Geometry check sheet. Reference: the model listing, model coordinates, mm. A direction names the side the tool comes from. Round coordinates to 2 decimals unless told otherwise and drop trailing zeros. Write each loop counter-clockwise with the first axis right and the second up, starting at its lowest first coordinate (ties: lowest second). Pieces come first, ordered by that corner, then holes. Notation, with made-up numbers: M 16.25,57 L 46.25,57 A25 cw 46.25,82 Z; hole C -18,1.25 d2. An arc over 180 degrees is marked long. Put each result on its own line as item: value. Start each with the question number.
(1) Gauge pin test, flat ends, axial feed: pin 1 (16.5 mm diameter, centred on x = -35, y = 6.5, fed in from -Z); pin 2 (7.5 mm diameter, centred on x = -35.5, y = 7, fed in from +Z); pin 3 (7.5 mm diameter, centred on y = 7.5, z = -22, fed in from -X). Record the tip position at first contact, or that the pin passes through.
(2) Material ranges on probe 1 along X at (y, z) = (26, -2); probe 2 along X at (y, z) = (12.5, -5); probe 3 along Z at (x, y) = (27, 28), recorded low to high.
(3) Tool access check on faces 1 (the flat face through (53, 7, -59.295)), 2 (the flat face through (-74.848, 27, -27)), 3 (the flat face through (52, 7, 5.705)). Record the directions out of +Z, -Z, +X, -X, +Y, -Y that give a thin tool (end or side, any length) a straight path to the whole face; none if there is none.
(4) Section check D-D on x = 34.5. Record the cut outline in (y, z), then the cut area to 3 significant figures.
(5) Section check B-B on y = 28. Record the cut outline in (x, z), then the cut area to 3 significant figures.
(6) Mould release check, pull along X, two halves, no side actions. Record for faces 4 (the flat face through (110.152, 25, -26)), 5 (the flat face through (52, 0, -27)), 6 (the flat face through (-84.848, 25, -26)), 7 (the flat face through (5.152, 7, -27)): pulls with the +X half, pulls with the -X half, needs draft (parallel to the pull), parting line crosses it, or undercut.
(7) Section check A-A on y = 9. Record the cut outline in (x, z).
(8) Section check C-C on z = -23.5. Record the cut outline in (x, y).
from build123d import *

# Parameters (mm, degrees)
BOSS_EXTRUDE2_DEPTH   = 15
BOSS_EXTRUDE2_2_DEPTH = 15
SKETCH2_W             = 195
SKETCH2_H             = 85
BOSS_EXTRUDE3_DEPTH   = 5
SKETCH3_W             = 195
SKETCH3_H             = 85
BOSS_EXTRUDE4_DEPTH   = 15


with BuildPart() as part:
    # Sketch1 → Boss-Extrude2 (new body)
    with BuildSketch(Plane(origin=(0, 0, 0), x_dir=(1, 0, 0), z_dir=(0, 1, 0))):
        with BuildLine():
            Line((-74.848214286, -3.705357143), (-74.848214286, 57.294642857))
            ThreePointArc((-74.848214286, 57.294642857), (-74.262427848, 58.70885642), (-72.848214286, 59.294642857))
            Line((-72.848214286, 59.294642857), (-6.848214286, 59.294642857))
            ThreePointArc((-6.848214286, 59.294642857), (-5.434000723, 58.70885642), (-4.848214286, 57.294642857))
            Line((-4.848214286, 57.294642857), (-4.848214286, -3.705357143))
            ThreePointArc((-4.848214286, -3.705357143), (-5.434000723, -5.119570705), (-6.848214286, -5.705357143))
            Line((-6.848214286, -5.705357143), (-72.848214286, -5.705357143))
            ThreePointArc((-72.848214286, -5.705357143), (-74.262427848, -5.119570705), (-74.848214286, -3.705357143))
        make_face()
    extrude(amount=BOSS_EXTRUDE2_DEPTH)



with BuildPart() as body_2:
    # Sketch1 → Boss-Extrude2 2 (new body)
    with BuildSketch(Plane(origin=(0, 0, 0), x_dir=(1, 0, 0), z_dir=(0, 1, 0))):
        with BuildLine():
            Line((100.151785714, -3.705357143), (100.151785714, 57.294642857))
            ThreePointArc((100.151785714, 57.294642857), (99.565999277, 58.70885642), (98.151785714, 59.294642857))
            Line((98.151785714, 59.294642857), (7.151785714, 59.294642857))
            ThreePointArc((7.151785714, 59.294642857), (5.737572152, 58.70885642), (5.151785714, 57.294642857))
            Line((5.151785714, 57.294642857), (5.151785714, -3.705357143))
            ThreePointArc((5.151785714, -3.705357143), (5.737572152, -5.119570705), (7.151785714, -5.705357143))
            Line((7.151785714, -5.705357143), (98.151785714, -5.705357143))
            ThreePointArc((98.151785714, -5.705357143), (99.565999277, -5.119570705), (100.151785714, -3.705357143))
        make_face()
    extrude(amount=BOSS_EXTRUDE2_2_DEPTH)


with BuildPart() as part_1:
    add(part.part)

    add(body_2.part)  # Boss-Extrude3 merges body 2
    # Sketch2 → Boss-Extrude3 (add)
    with BuildSketch(Plane(origin=(0, 15, 0), x_dir=(1, 0, 0), z_dir=(0, 1, 0))):
        with Locations((12.651785714, 26.794642857)):
            Rectangle(SKETCH2_W, SKETCH2_H)
    extrude(amount=BOSS_EXTRUDE3_DEPTH)

    # Sketch3 → Boss-Extrude4 (add)
    with BuildSketch(Plane(origin=(0, 20, 0), x_dir=(1, 0, 0), z_dir=(0, 1, 0))):
        with Locations((12.651785714, 26.794642857)):
            Rectangle(SKETCH3_W, SKETCH3_H)
        with BuildLine():
            Line((-74.848214286, 57.294642857), (-74.848214286, -3.705357143))
            ThreePointArc((-74.848214286, -3.705357143), (-74.262427848, -5.119570705), (-72.848214286, -5.705357143))
            Line((-72.848214286, -5.705357143), (98.151785714, -5.705357143))
            ThreePointArc((98.151785714, -5.705357143), (99.565999277, -5.119570705), (100.151785714, -3.705357143))
            Line((100.151785714, -3.705357143), (100.151785714, 57.294642857))
            ThreePointArc((100.151785714, 57.294642857), (99.565999277, 58.70885642), (98.151785714, 59.294642857))
            Line((98.151785714, 59.294642857), (-72.848214286, 59.294642857))
            ThreePointArc((-72.848214286, 59.294642857), (-74.262427848, 58.70885642), (-74.848214286, 57.294642857))
        make_face(mode=Mode.SUBTRACT)
    extrude(amount=BOSS_EXTRUDE4_DEPTH)


solid = part_1.part
Answers follow:
1. pin 1: stops at z = -59.29
1. pin 2: stops at z = 5.71
1. pin 3: stops at x = -74.85
2. probe 1: x = -84.85 to -74.85, 100.15 to 110.15
2. probe 2: x = -74.85 to -4.85, 5.15 to 100.15
2. probe 3: z = -69.29 to -59.29, 5.71 to 15.71
3. face 1: -Z, +X, -X, -Y
3. face 2: +Y
3. face 3: +Z, +X, -X, -Y
4. outline: M 0,-59.29 L 15,-59.29 L 15,-69.29 L 35,-69.29 L 35,-59.29 L 20,-59.29 L 20,5.71 L 35,5.71 L 35,15.71 L 15,15.71 L 15,5.71 L 0,5.71 Z
4. area: 1,700 mm^2
5. outline: M -84.85,-69.29 L 110.15,-69.29 L 110.15,15.71 L -84.85,15.71 Z; hole M -74.85,-57.29 A2 ccw -72.85,-59.29 L 98.15,-59.29 A2 ccw 100.15,-57.29 L 100.15,3.71 A2 ccw 98.15,5.71 L -72.85,5.71 A2 ccw -74.85,3.71 Z
5. area: 5,200 mm^2
6. face 4: pulls with the +X half
6. face 5: needs draft
6. face 6: pulls with the -X half
6. face 7: undercut
7. outline: M -74.85,-57.29 A2 ccw -72.85,-59.29 L -6.85,-59.29 A2 ccw -4.85,-57.29 L -4.85,3.71 A2 ccw -6.85,5.71 L -72.85,5.71 A2 ccw -74.85,3.71 Z; M 5.15,-57.29 A2 ccw 7.15,-59.29 L 98.15,-59.29 A2 ccw 100.15,-57.29 L 100.15,3.71 A2 ccw 98.15,5.71 L 7.15,5.71 A2 ccw 5.15,3.71 Z
8. outline: M -84.85,15 L -74.85,15 L -74.85,0 L -4.85,0 L -4.85,15 L 5.15,15 L 5.15,0 L 100.15,0 L 100.15,15 L 110.15,15 L 110.15,35 L 100.15,35 L 100.15,20 L -74.85,20 L -74.85,35 L -84.85,35 Z
